```python
from build123d import *

# Parameters (mm, degrees)
SKETCH1_W                = 8
SKETCH1_H                = 41.5
SKETCH1_R                = 1.75
BOSS_EXTRUDE2_DEPTH      = 2
CIRPATTERN1_COUNT        = 3
BOSS_EXTRUDE4_DEPTH      = 4
FILLET4_R                = 1
FILLET5_R                = 1
CIRPATTERN2_COUNT        = 3
FILLET4_OF_CIRPATTERN2_R = 1
FILLET5_OF_CIRPATTERN2_R = 1
FILLET6_R                = 10


with BuildPart() as part:
    # Sketch1 → Boss-Extrude2 (new body)
    with BuildSketch(Plane(origin=(0, 0, 0), x_dir=(1, 0, 0), z_dir=(0, 1, 0))):
        with Locations((4, 20.75)):
            Rectangle(SKETCH1_W, SKETCH1_H)
        with Locations(Location((4, 37.5, 0), (0, 0, 270))):
            Circle(SKETCH1_R, mode=Mode.SUBTRACT)
    boss_extrude2 = extrude(amount=BOSS_EXTRUDE2_DEPTH)

    # CirPattern1: Boss-Extrude2 ×3 about axis
    cirpattern1_axis = Axis((4, 0, 0), (0, 1, 0))
    for i in range(1, CIRPATTERN1_COUNT):
        add(boss_extrude2.rotate(cirpattern1_axis, i * 360 / CIRPATTERN1_COUNT))

    # Sketch8 → Boss-Extrude4 (add, symmetric)
    with BuildSketch(Plane(origin=(4, 0, 0), x_dir=(0, 0, -1), z_dir=(1, 0, 0))):
        with BuildLine():
            Line((41.5, 0), (42.621101534, 0))
            ThreePointArc((42.621101534, 0), (43.575288985, 0.405725605), (43.945070079, 1.374409713))
            ThreePointArc((43.945070079, 1.374409713), (44.287115262, 4.314035864), (45.5, 7.013537193))
            Line((45.5, 7.013537193), (43.885890552, 8.06067472))
            Line((43.885890552, 8.06067472), (42.771717246, 2.127015587))
            Line((42.771717246, 2.127015587), (41.5, 2))
            Line((41.5, 2), (41.5, 0))
        make_face()
    boss_extrude4 = extrude(amount=BOSS_EXTRUDE4_DEPTH, both=True)

    # Fillet4
    # the kernel refuses this fillet: 1 mm, written as the material it takes off along each edge
    with BuildSketch(Plane(origin=(11.730116112, 8.06067472, -43.885890552), x_dir=(0, -0.9828237835068792, 0.1845464997587953), z_dir=(-1, 0, 0))) as fillet4_piece_1:
        with BuildLine():
            CenterArc((FILLET4_R * 1.49204644486, -FILLET4_R), FILLET4_R, 90, 112.338398351)
            Line((FILLET4_R * 0.567091237268, -FILLET4_R * 1.38007612915), (0, 0))
            Line((0, 0), (FILLET4_R * 1.49204644486, 0))
        make_face()
    extrude(amount=15.460232224, mode=Mode.SUBTRACT)
    with BuildSketch(Plane(origin=(-2.382872769, 7.013537193, -45.5), x_dir=(0, 0.5442451052621637, 0.8389262574256311), z_dir=(1, 0, 0))) as fillet4_piece_2:
        with BuildLine():
            CenterArc((0.953149108, 1), FILLET4_R, 185.36479385, 84.63520615)
            ThreePointArc((-0.042470495, 0.906503441), (-0.010623444, 0.453748893), (0, 0))
            Line((0, 0), (0.953149108, 0))
        make_face()
    extrude(amount=12.765745538, mode=Mode.SUBTRACT)

    # Fillet5
    # the kernel refuses this fillet: 1 mm, written as the material it adds along each edge
    with BuildSketch(Plane(origin=(8, 2, -41.5), x_dir=(0, 0, 1), z_dir=(-1, 0, 0))) as fillet5_piece_1:
        with BuildLine():
            CenterArc((FILLET5_R * 0.0498146888591, FILLET5_R), FILLET5_R, 264.296371881, 5.703628119)
            Line((-FILLET5_R * 0.0495680702218, FILLET5_R * 0.00495072122158), (0, 0))
            Line((0, 0), (FILLET5_R * 0.0498146888591, 0))
        make_face()
    extrude(amount=8)
    with BuildSketch(Plane(origin=(8, 2.127015587, -42.771717246), x_dir=(0, 0.9828237835068792, -0.18454649975879509), z_dir=(-1, 0, 0))) as fillet5_piece_2:
        with BuildLine():
            CenterArc((FILLET5_R * 0.748935389987, -FILLET5_R), FILLET5_R, 90, 73.66167838)
            Line((-FILLET5_R * 0.210681966633, -FILLET5_R * 0.718691399219), (0, 0))
            Line((0, 0), (FILLET5_R * 0.748935389987, 0))
        make_face()
    extrude(amount=8)

    # CirPattern2: Boss-Extrude4 ×3 about axis
    cirpattern2_axis = Axis((4, 0, 0), (0, 1, 0))
    for i in range(1, CIRPATTERN2_COUNT):
        add(boss_extrude4.rotate(cirpattern2_axis, i * 360 / CIRPATTERN2_COUNT))

    # Fillet4 of CirPattern2
    # the kernel refuses this fillet: 1 mm, written as the material it takes off along each edge
    with BuildSketch(Plane(origin=(-37.871354141, 8.06067472, 15.248468348), x_dir=(-0.7265314508324002, -0.5442451052621637, 0.4194631287128154), z_dir=(0.49999999999999983, 0, 0.8660254037844388))) as fillet4_of_cirpattern2_piece_1:
        with BuildLine():
            CenterArc((FILLET4_OF_CIRPATTERN2_R * 1.49204644486, FILLET4_OF_CIRPATTERN2_R), FILLET4_OF_CIRPATTERN2_R, 157.661601649, 112.338398351)
            Line((FILLET4_OF_CIRPATTERN2_R * 0.567091237268, FILLET4_OF_CIRPATTERN2_R * 1.38007612915), (0, 0))
            Line((0, 0), (FILLET4_OF_CIRPATTERN2_R * 1.49204644486, 0))
        make_face()
    extrude(amount=15.460232224, mode=Mode.SUBTRACT)
    with BuildSketch(Plane(origin=(-32.212719488, 7.013537193, 28.277729967), x_dir=(0.43681230013054545, -0.8634774766062033, -0.2521936990657099), z_dir=(-0.49999999999999983, 0, -0.8660254037844388))) as fillet4_of_cirpattern2_piece_2:
        with BuildLine():
            CenterArc((0.954297344, -0.9989043), FILLET4_OF_CIRPATTERN2_R, 92.682396925, 84.63520615)
            Line((-0.044606957, -0.952104742), (0, 0))
            ThreePointArc((0, 0), (0.453748893, -0.010623444), (0.907497786, 0))
        make_face()
    extrude(amount=12.765745538, mode=Mode.SUBTRACT)
    with BuildSketch(Plane(origin=(38.141238029, 8.06067472, 28.637422203), x_dir=(-0.15982195697061236, -0.9828237835068798, -0.09227324987939595), z_dir=(0.5000000000000004, 0, -0.8660254037844384))) as fillet4_of_cirpattern2_piece_3:
        with BuildLine():
            CenterArc((FILLET4_OF_CIRPATTERN2_R * 1.49204644486, -FILLET4_OF_CIRPATTERN2_R), FILLET4_OF_CIRPATTERN2_R, 90, 112.338398351)
            Line((FILLET4_OF_CIRPATTERN2_R * 0.567091237268, -FILLET4_OF_CIRPATTERN2_R * 1.38007612915), (0, 0))
            Line((0, 0), (FILLET4_OF_CIRPATTERN2_R * 1.49204644486, 0))
        make_face()
    extrude(amount=15.460232224, mode=Mode.SUBTRACT)
    with BuildSketch(Plane(origin=(46.595592257, 7.013537193, 17.222270033), x_dir=(-0.7265314508324002, 0.5442451052621633, -0.4194631287128161), z_dir=(-0.5000000000000004, 0, 0.8660254037844384))) as fillet4_of_cirpattern2_piece_4:
        with BuildLine():
            CenterArc((0.953149108, 1), FILLET4_OF_CIRPATTERN2_R, 185.36479385, 84.63520615)
            ThreePointArc((-0.042470495, 0.906503441), (-0.010623444, 0.453748893), (0, 0))
            Line((0, 0), (0.953149108, 0))
        make_face()
    extrude(amount=12.765745538, mode=Mode.SUBTRACT)

    # Fillet5 of CirPattern2
    # the kernel refuses this fillet: 1 mm, written as the material it adds along each edge
    with BuildSketch(Plane(origin=(-33.940054257, 2, 17.285898385), x_dir=(0.8660254037844387, 0, -0.4999999999999998), z_dir=(0.49999999999999983, 0, 0.8660254037844388)), Plane(origin=(37.940054257, 2, 24.214101615), x_dir=(-0.8660254037844384, 0, -0.5000000000000004), z_dir=(0.5000000000000004, 0, -0.8660254037844384))) as fillet5_of_cirpattern2_piece_1:
        with BuildLine():
            CenterArc((FILLET5_OF_CIRPATTERN2_R * 0.0498146888591, FILLET5_OF_CIRPATTERN2_R), FILLET5_OF_CIRPATTERN2_R, 264.296371881, 5.703628119)
            Line((-FILLET5_OF_CIRPATTERN2_R * 0.0495680702218, FILLET5_OF_CIRPATTERN2_R * 0.00495072122158), (0, 0))
            Line((0, 0), (FILLET5_OF_CIRPATTERN2_R * 0.0498146888591, 0))
        make_face()
    extrude(amount=8)
    with BuildSketch(Plane(origin=(-35.041393699, 2.127015587, 17.921757008), x_dir=(0.861737953439498, -0.0993827590809451, -0.4975246393892111), z_dir=(0.49999999999999983, 0, 0.8660254037844388)), Plane(origin=(39.041393699, 2.127015587, 24.849960238), x_dir=(-0.8617379534394976, -0.09938275908094509, -0.49752463938921165), z_dir=(0.5000000000000004, 0, -0.8660254037844384))) as fillet5_of_cirpattern2_piece_2:
        with BuildLine():
            CenterArc((FILLET5_OF_CIRPATTERN2_R * 0.748935389987, FILLET5_OF_CIRPATTERN2_R), FILLET5_OF_CIRPATTERN2_R, 196.33832162, 73.66167838)
            Line((-FILLET5_OF_CIRPATTERN2_R * 0.210681966633, FILLET5_OF_CIRPATTERN2_R * 0.718691399219), (0, 0))
            Line((0, 0), (FILLET5_OF_CIRPATTERN2_R * 0.748935389987, 0))
        make_face()
    extrude(amount=8)

    # Fillet6
    fillet6_edges = [part.edges().sort_by_distance(p)[0] for p in [
        (8, 1, -2.309401077),
        (0, 1, -2.309401077),
        (4, 1, 4.618802154),
    ]]
    fillet(fillet6_edges, radius=FILLET6_R)


solid = part.part
```
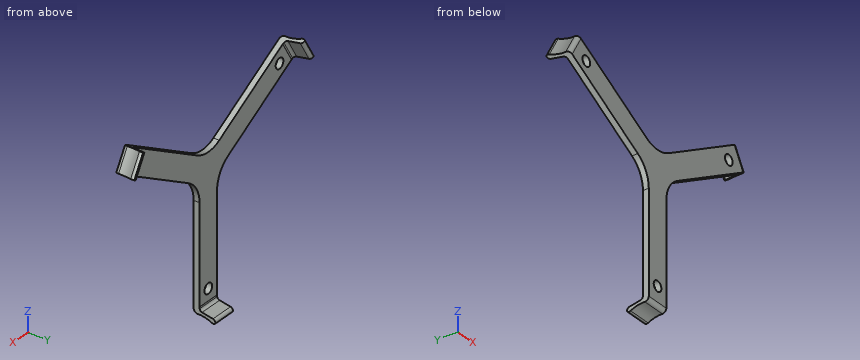
Input: part model. Units: mm. Frame: model coordinates. Coordinates: 2 decimals unless noted, no trailing zeros. Loops run counter-clockwise (first coordinate to the right, second up) from the corner with the lowest first, then second, coordinate; pieces in that order, holes last. Notation, with made-up numbers: M 36.5,67 L 67.5,67 A10 cw 67.5,81 Z; hole C 32,13 d9. An arc over 180 degrees is marked long. Answer in a Markdown table with one row per item.
1. Section A-A, the plane z = -37.5. Output: boundary loops of the cut face in (x, y).
Response:
| item | result |
|---|---|
| outline | M 0,0 L 2.25,0 L 2.25,2 L 0,2 Z; M 5.75,0 L 8,0 L 8,2 L 5.75,2 Z |
2. First-contact query: pin 1 (5.5 mm diameter, centred on x = -28.48, z = 18.75, fed in from +Y); pin 2 (3 mm diameter, centred on x = 5.5, y = 1, fed in from +Z). Flat tips, straight axial feed; report the tip coordinate or a pass-through.
Response:
| item | result |
|---|---|
| pin 1 | stops at y = 2 |
| pin 2 | stops at z = 6.63 |
3. Section B-B, the plane x = 37. Output: boundary loops of the cut face in (y, z), then the cut area to 3 significant figures.
Response:
| item | result |
|---|---|
| outline | M 0,14.43 L 2,14.43 L 2,17.08 L 0,17.08 Z; M 0,20.42 L 2,20.42 L 2,23.67 L 0,23.67 Z |
| area | 11.8 mm2 |
4. Section D-D, the plane z = -11. Output: boundary loops of the cut face in (x, y), then the cut area to 3 significant figures.
Response:
| item | result |
|---|---|
| outline | M 0,0 L 8,0 L 8,2 L 0,2 Z |
| area | 16.0 mm2 |
5. Material intervals for line 1 (X direction, y = 1.3, z = -37.5); line 2 (X direction, y = 1.4, z = 18.75); line 3 (X direction, y = 0.8, z = 18.75), sorted ascending.
Response:
| item | result |
|---|---|
| line 1 | x = 0 to 2.25, 5.75 to 8 |
| line 2 | x = -35.92 to -30.23, -26.73 to -20.48, 28.48 to 34.73, 38.23 to 43.92 |
| line 3 | x = -35.79 to -30.23, -26.73 to -20.48, 28.48 to 34.73, 38.23 to 43.79 |
6. Section C-C, the plane y = 4.5. Output: boundary loops of the cut face in (x, z).
Response:
| item | result |
|---|---|
| outline | M -36.4,18.71 L -35.43,18.14 L -31.43,25.07 L -32.4,25.63 Z; M 0,-44.34 L 8,-44.34 L 8,-43.22 L 0,-43.22 Z; M 39.43,25.07 L 43.43,18.14 L 44.4,18.71 L 40.4,25.63 Z |
